Can you work these out from the model? Positions are in its coordinate system, mm. A direction names the side the tool comes from. Coordinates: 2 decimals unless noted, no trailing zeros. Order: outer loops, then holes, each group sorted by start corner. A loop starts at its lowest first (then second) coordinate and runs counter-clockwise, first axis right, second up. Notation, with made-up numbers: (0.25, 24.5) -> (17.25, 24.5) arc R35 ccw to (17.25, 59.5) -> close; hole circle Ø7 at (76.5, -2). An arc over 180 degrees is marked (long way). Return JSON: item names as keys, results as strings. Group by question number.
1) If we section it at B-B, the plane x = 63.5: Please give me the cut outline in (y, z), then the cut area to 3 significant figures.
2) If we section it at C-C, the plane x = 118: Please give me the cut outline in (y, z).
3) If we section it at D-D, the plane z = 2.4: State how many separate pieces and enclosed holes the cut face has, then the cut area to 3 significant figures.
4) For faces 4 (the flat face through (139.664, 53, 2)), 5 (the flat face through (0, 58, 2)), which set-ups out of +Z, -Z, +X, -X, +Y, -Y let a thin tool reach every point of the face, with its end or its side?
5) For pin 1 (13 mm diameter, centred on x = 18, y = 18, fed in from -Z), with a flat end and sliding along its axis, tell me the tip position at first contact or that it passes through.
6) Thinking about a two-plate mould opening in Y: for faces 1 (the flat face through (159, 58, 2)), 2 (the flat face through (78, 117, 2)), 3 (the flat face through (71, 14.5, 2)), which applies, +Y half, -Y half, draft (parallel to the pull), parting line (faces both ways), or undercut?
7) If we section it at A-A, the plane y = 77: Please give me the cut outline in (x, z), then the cut area to 3 significant figures.
8) If I drill on probe 1 along Y at (x, z) = (40, 0.6); probe 2 along X at (y, z) = (75, 2); probe 3 along X at (y, z) = (40, 3.75), over which ranges is the centre line in solid material (lowest first)? Write a range as from..to.
from build123d import *

# Parameters (mm, degrees)
ESQUISSE1_W                  = 159
ESQUISSE1_H                  = 117
BOSS_EXTRU_1_DEPTH           = 4
ESQUISSE3_W                  = 101.76
ESQUISSE3_H                  = 76.32
ENL_V_MAT_EXTRU_2_DEPTH      = 4
ESQUISSE9_W                  = 118
ESQUISSE9_H                  = 88.9
ENL_V_MAT_EXTRU_5_DEPTH      = 3
ESQUISSE4_R                  = 4
ENL_V_MAT_EXTRU_3_DEPTH      = 4
ESQUISSE10_R                 = 3
ENL_V_MAT_EXTRU_6_DEPTH      = 4
ENL_V_MAT_EXTRU_7_DEPTH      = 8.5
ENL_V_MAT_EXTRU_7_DEPTH_BACK = 1.5
ESQUISSE11_R                 = 1.75


with BuildPart() as part:
    # Esquisse1 → Boss.-Extru.1 (new body)
    with BuildSketch(Plane.XY):
        with Locations((79.5, 58.5)):
            Rectangle(ESQUISSE1_W, ESQUISSE1_H)
    extrude(amount=BOSS_EXTRU_1_DEPTH)

    # Esquisse3 → Enlèv. mat.-Extru.2 (cut)
    with BuildSketch(Plane.XY.offset(4)):
        with Locations((79.5, 68.84)):
            Rectangle(ESQUISSE3_W, ESQUISSE3_H)
    extrude(amount=-ENL_V_MAT_EXTRU_2_DEPTH, mode=Mode.SUBTRACT)

    # Esquisse9 → Enlèv. mat.-Extru.5 (cut)
    with BuildSketch(Plane(origin=(0, 0, 0), x_dir=(-1, 0, 0), z_dir=(0, 0, -1))):
        with Locations((-79.163992303, 67.176625881)):
            Rectangle(ESQUISSE9_W, ESQUISSE9_H)
    extrude(amount=-ENL_V_MAT_EXTRU_5_DEPTH, mode=Mode.SUBTRACT)

    # Esquisse4 → Enlèv. mat.-Extru.3 (cut)
    with BuildSketch(Plane.XY.offset(4)):
        with Locations((141, 18)):
            Circle(ESQUISSE4_R)
        with Locations((18, 18)):
            Circle(ESQUISSE4_R)
    extrude(amount=-ENL_V_MAT_EXTRU_3_DEPTH, mode=Mode.SUBTRACT)

    # Esquisse10 → Enlèv. mat.-Extru.6 (cut)
    with BuildSketch(Plane(origin=(0, 0, 0), x_dir=(-1, 0, 0), z_dir=(0, 0, -1))):
        with Locations((-10.163992303, 90)):
            Circle(ESQUISSE10_R)
        with Locations((-10.163992303, 67)):
            Circle(ESQUISSE10_R)
        with BuildLine():
            Line((-124, 21.5), (-115, 21.5))
            ThreePointArc((-115, 21.5), (-114.292893219, 21.207106781), (-114, 20.5))
            Line((-114, 20.5), (-114, 15.5))
            ThreePointArc((-114, 15.5), (-114.292893219, 14.792893219), (-115, 14.5))
            Line((-115, 14.5), (-124, 14.5))
            ThreePointArc((-124, 14.5), (-124.707106781, 14.792893219), (-125, 15.5))
            Line((-125, 15.5), (-125, 20.5))
            ThreePointArc((-125, 20.5), (-124.707106781, 21.207106781), (-124, 21.5))
        make_face()
        with BuildLine():
            Line((-108, 21.5), (-99, 21.5))
            ThreePointArc((-99, 21.5), (-98.292893219, 21.207106781), (-98, 20.5))
            Line((-98, 20.5), (-98, 15.5))
            ThreePointArc((-98, 15.5), (-98.292893219, 14.792893219), (-99, 14.5))
            Line((-99, 14.5), (-108, 14.5))
            ThreePointArc((-108, 14.5), (-108.707106781, 14.792893219), (-109, 15.5))
            Line((-109, 15.5), (-109, 20.5))
            ThreePointArc((-109, 20.5), (-108.707106781, 21.207106781), (-108, 21.5))
        make_face()
        with BuildLine():
            Line((-92, 21.5), (-83, 21.5))
            ThreePointArc((-83, 21.5), (-82.292893219, 21.207106781), (-82, 20.5))
            Line((-82, 20.5), (-82, 15.5))
            ThreePointArc((-82, 15.5), (-82.292893219, 14.792893219), (-83, 14.5))
            Line((-83, 14.5), (-92, 14.5))
            ThreePointArc((-92, 14.5), (-92.707106781, 14.792893219), (-93, 15.5))
            Line((-93, 15.5), (-93, 20.5))
            ThreePointArc((-93, 20.5), (-92.707106781, 21.207106781), (-92, 21.5))
        make_face()
        with BuildLine():
            Line((-76, 21.5), (-67, 21.5))
            ThreePointArc((-67, 21.5), (-66.292893219, 21.207106781), (-66, 20.5))
            Line((-66, 20.5), (-66, 15.5))
            ThreePointArc((-66, 15.5), (-66.292893219, 14.792893219), (-67, 14.5))
            Line((-67, 14.5), (-76, 14.5))
            ThreePointArc((-76, 14.5), (-76.707106781, 14.792893219), (-77, 15.5))
            Line((-77, 15.5), (-77, 20.5))
            ThreePointArc((-77, 20.5), (-76.707106781, 21.207106781), (-76, 21.5))
        make_face()
        with BuildLine():
            Line((-60, 21.5), (-51, 21.5))
            ThreePointArc((-51, 21.5), (-50.292893219, 21.207106781), (-50, 20.5))
            Line((-50, 20.5), (-50, 15.5))
            ThreePointArc((-50, 15.5), (-50.292893219, 14.792893219), (-51, 14.5))
            Line((-51, 14.5), (-60, 14.5))
            ThreePointArc((-60, 14.5), (-60.707106781, 14.792893219), (-61, 15.5))
            Line((-61, 15.5), (-61, 20.5))
            ThreePointArc((-61, 20.5), (-60.707106781, 21.207106781), (-60, 21.5))
        make_face()
        with BuildLine():
            Line((-44, 21.5), (-35, 21.5))
            ThreePointArc((-35, 21.5), (-34.292893219, 21.207106781), (-34, 20.5))
            Line((-34, 20.5), (-34, 15.5))
            ThreePointArc((-34, 15.5), (-34.292893219, 14.792893219), (-35, 14.5))
            Line((-35, 14.5), (-44, 14.5))
            ThreePointArc((-44, 14.5), (-44.707106781, 14.792893219), (-45, 15.5))
            Line((-45, 15.5), (-45, 20.5))
            ThreePointArc((-45, 20.5), (-44.707106781, 21.207106781), (-44, 21.5))
        make_face()
        with BuildLine():
            Line((-147.663992303, 107), (-142.663992303, 107))
            ThreePointArc((-142.663992303, 107), (-141.956885522, 106.707106781), (-141.663992303, 106))
            Line((-141.663992303, 106), (-141.663992303, 86))
            ThreePointArc((-141.663992303, 86), (-141.956885522, 85.292893219), (-142.663992303, 85))
            Line((-142.663992303, 85), (-147.663992303, 85))
            ThreePointArc((-147.663992303, 85), (-148.371099084, 85.292893219), (-148.663992303, 86))
            Line((-148.663992303, 86), (-148.663992303, 106))
            ThreePointArc((-148.663992303, 106), (-148.371099084, 106.707106781), (-147.663992303, 107))
        make_face()
        with BuildLine():
            Line((-149.663992303, 80), (-140.663992303, 80))
            ThreePointArc((-140.663992303, 80), (-139.956885522, 79.707106781), (-139.663992303, 79))
            Line((-139.663992303, 79), (-139.663992303, 74))
            ThreePointArc((-139.663992303, 74), (-139.956885522, 73.292893219), (-140.663992303, 73))
            Line((-140.663992303, 73), (-149.663992303, 73))
            ThreePointArc((-149.663992303, 73), (-150.371099084, 73.292893219), (-150.663992303, 74))
            Line((-150.663992303, 74), (-150.663992303, 79))
            ThreePointArc((-150.663992303, 79), (-150.371099084, 79.707106781), (-149.663992303, 80))
        make_face()
        with BuildLine():
            Line((-149.663992303, 68), (-140.663992303, 68))
            ThreePointArc((-140.663992303, 68), (-139.956885522, 67.707106781), (-139.663992303, 67))
            Line((-139.663992303, 67), (-139.663992303, 62))
            ThreePointArc((-139.663992303, 62), (-139.956885522, 61.292893219), (-140.663992303, 61))
            Line((-140.663992303, 61), (-149.663992303, 61))
            ThreePointArc((-149.663992303, 61), (-150.371099084, 61.292893219), (-150.663992303, 62))
            Line((-150.663992303, 62), (-150.663992303, 67))
            ThreePointArc((-150.663992303, 67), (-150.371099084, 67.707106781), (-149.663992303, 68))
        make_face()
        with BuildLine():
            Line((-149.663992303, 56), (-140.663992303, 56))
            ThreePointArc((-140.663992303, 56), (-139.956885522, 55.707106781), (-139.663992303, 55))
            Line((-139.663992303, 55), (-139.663992303, 50))
            ThreePointArc((-139.663992303, 50), (-139.956885522, 49.292893219), (-140.663992303, 49))
            Line((-140.663992303, 49), (-149.663992303, 49))
            ThreePointArc((-149.663992303, 49), (-150.371099084, 49.292893219), (-150.663992303, 50))
            Line((-150.663992303, 50), (-150.663992303, 55))
            ThreePointArc((-150.663992303, 55), (-150.371099084, 55.707106781), (-149.663992303, 56))
        make_face()
        with BuildLine():
            Line((-149.663992303, 44), (-140.663992303, 44))
            ThreePointArc((-140.663992303, 44), (-139.956885522, 43.707106781), (-139.663992303, 43))
            Line((-139.663992303, 43), (-139.663992303, 38))
            ThreePointArc((-139.663992303, 38), (-139.956885522, 37.292893219), (-140.663992303, 37))
            Line((-140.663992303, 37), (-149.663992303, 37))
            ThreePointArc((-149.663992303, 37), (-150.371099084, 37.292893219), (-150.663992303, 38))
            Line((-150.663992303, 38), (-150.663992303, 43))
            ThreePointArc((-150.663992303, 43), (-150.371099084, 43.707106781), (-149.663992303, 44))
        make_face()
        with BuildLine():
            Line((-15.663992303, 107), (-10.663992303, 107))
            ThreePointArc((-10.663992303, 107), (-9.956885522, 106.707106781), (-9.663992303, 106))
            Line((-9.663992303, 106), (-9.663992303, 97))
            ThreePointArc((-9.663992303, 97), (-9.956885522, 96.292893219), (-10.663992303, 96))
            Line((-10.663992303, 96), (-15.663992303, 96))
            ThreePointArc((-15.663992303, 96), (-16.371099084, 96.292893219), (-16.663992303, 97))
            Line((-16.663992303, 97), (-16.663992303, 106))
            ThreePointArc((-16.663992303, 106), (-16.371099084, 106.707106781), (-15.663992303, 107))
        make_face()
        with BuildLine():
            Line((-15.663992303, 84), (-10.663992303, 84))
            ThreePointArc((-10.663992303, 84), (-9.956885522, 83.707106781), (-9.663992303, 83))
            Line((-9.663992303, 83), (-9.663992303, 74))
            ThreePointArc((-9.663992303, 74), (-9.956885522, 73.292893219), (-10.663992303, 73))
            Line((-10.663992303, 73), (-15.663992303, 73))
            ThreePointArc((-15.663992303, 73), (-16.371099084, 73.292893219), (-16.663992303, 74))
            Line((-16.663992303, 74), (-16.663992303, 83))
            ThreePointArc((-16.663992303, 83), (-16.371099084, 83.707106781), (-15.663992303, 84))
        make_face()
    extrude(amount=-ENL_V_MAT_EXTRU_6_DEPTH, mode=Mode.SUBTRACT)

    # Esquisse11 → Enlèv. mat.-Extru.7 (cut, two sides: drawn at the far end of the back side and taken through both)
    with BuildSketch(Plane.ZY.offset(-148.663992303).offset(-ENL_V_MAT_EXTRU_7_DEPTH_BACK)):
        with Locations((0, 96)):
            Circle(ESQUISSE11_R)
    extrude(amount=ENL_V_MAT_EXTRU_7_DEPTH + ENL_V_MAT_EXTRU_7_DEPTH_BACK, mode=Mode.SUBTRACT)


solid = part.part
Result sheet:
{
 "1": {"outline": "(0, 0) -> (22.73, 0) -> (22.73, 3) -> (30.68, 3) -> (30.68, 4) -> (0, 4) -> close; (107, 3) -> (111.63, 3) -> (111.63, 0) -> (117, 0) -> (117, 4) -> (107, 4) -> close", "area": "125 mm2"},
 "2": {"outline": "(0, 0) -> (14.5, 0) -> (14.5, 4) -> (0, 4) -> close; (21.5, 0) -> (22.73, 0) -> (22.73, 3) -> (30.68, 3) -> (30.68, 4) -> (21.5, 4) -> close; (107, 3) -> (111.63, 3) -> (111.63, 0) -> (117, 0) -> (117, 4) -> (107, 4) -> close"},
 "3": {"separate pieces": "1", "enclosed holes": "18", "area": "6,890 mm2"},
 "4": {"face 4": "+Z, -Z", "face 5": "+Z, -Z, -X, +Y, -Y"},
 "5": {"pin 1": "stops at z = 0"},
 "6": {"face 1": "draft", "face 2": "+Y half", "face 3": "undercut"},
 "7": {"outline": "(0, 0) -> (9.66, 0) -> (9.66, 4) -> (0, 4) -> close; (16.66, 0) -> (20.16, 0) -> (20.16, 3) -> (28.62, 3) -> (28.62, 4) -> (16.66, 4) -> close; (130.38, 3) -> (138.16, 3) -> (138.16, 0) -> (139.66, 0) -> (139.66, 4) -> (130.38, 4) -> close; (150.66, 0) -> (159, 0) -> (159, 4) -> (150.66, 4) -> close", "area": "108 mm2"},
 "8": {"probe 1": "y = 0..14.5, 21.5..22.73, 111.63..117", "probe 2": "x = 0..9.66, 16.66..20.16, 138.16..139.66, 150.66..159", "probe 3": "x = 0..28.62, 130.38..139.66, 150.66..159"}
}
